Could you check a few things on this model? Use its own coordinates, in mm. Face numbers are marked on the shaded views. A direction names the side the tool comes from. Give positions to 0.01 mm unless a question says otherwise; leave off trailing zeros. Write each loop counter-clockwise with the first axis right and the second up, starting at its lowest first coordinate (ties: lowest second). Pieces come first, ordered by that corner, then holes. Notation, with made-up numbers: M -0.75,10.5 L 12.25,10.5 A11 ccw 12.25,14.5 Z; hole C -32.5,71.25 d8. An arc over 180 degrees is marked long. One line per item, written item: value.
```python
from build123d import *

# Parameters (mm, degrees)
BOSS_EXTRUDE2_DEPTH = 25.4
CUT_EXTRUDE7_START  = -1
SKETCH5_5_R         = 1.89865
CUT_EXTRUDE7_DEPTH  = 11.8425
SKETCH8_R           = 5.70865
SKETCH8_R_2         = 1.89865
BOSS_EXTRUDE4_DEPTH = 5.08
CUT_EXTRUDE8_START  = 5.08
SKETCH8_3_R         = 5.70865
SKETCH8_3_R_2       = 1.89865
CUT_EXTRUDE8_DEPTH  = 5.7625001
CUT_EXTRUDE3_DEPTH  = 26.4000001
FILLET3_R           = 1.905


with BuildPart() as part:
    # Sketch4 → Boss-Extrude2 (new body)
    with BuildSketch(Plane(origin=(-23.495, 41.0349954, 0), x_dir=(0, 0, 1), z_dir=(-1, 0, 0))):
        with BuildLine():
            ThreePointArc((0, 16.227532365), (9.8425, 0), (0, -16.227532365))
            Line((0, -16.227532365), (0, -10.16))
            ThreePointArc((0, -10.16), (4.7625, 0), (0, 10.16))
            Line((0, 10.16), (0, 16.227532365))
        make_face()
    extrude(amount=-BOSS_EXTRUDE2_DEPTH)

    # Sketch5_5 → Cut-Extrude7 (cut)
    with BuildSketch(Plane.XY.offset(CUT_EXTRUDE7_START)):
        with Locations((-10.795, 55.2907454)):
            Circle(SKETCH5_5_R)
    cut_extrude7 = extrude(amount=CUT_EXTRUDE7_DEPTH, mode=Mode.SUBTRACT)

    # Sketch8 → Boss-Extrude4 (add)
    with BuildSketch(Plane.XY):
        with Locations((-10.795, 55.2907454)):
            Circle(SKETCH8_R)
        with Locations((-10.795, 55.2907454)):
            Circle(SKETCH8_R_2, mode=Mode.SUBTRACT)
    boss_extrude4 = extrude(amount=BOSS_EXTRUDE4_DEPTH)

    # Sketch8_3 → Cut-Extrude8 (cut, through all)
    with BuildSketch(Plane.XY.offset(CUT_EXTRUDE8_START)):
        with Locations((-10.795, 55.2907454)):
            Circle(SKETCH8_3_R)
        with Locations((-10.795, 55.2907454)):
            Circle(SKETCH8_3_R_2, mode=Mode.SUBTRACT)
    cut_extrude8 = extrude(amount=CUT_EXTRUDE8_DEPTH, mode=Mode.SUBTRACT)

    # Mirror1: Cut-Extrude7, Boss-Extrude4, Cut-Extrude8 across plane
    add(cut_extrude7.mirror(Plane.ZX.offset(41.0349954)), mode=Mode.SUBTRACT)
    add(boss_extrude4.mirror(Plane.ZX.offset(41.0349954)))
    add(cut_extrude8.mirror(Plane.ZX.offset(41.0349954)), mode=Mode.SUBTRACT)

    # Sketch4_3 → Cut-Extrude3 (cut, through all)
    with BuildSketch(Plane(origin=(-23.495, 41.0349954, 0), x_dir=(0, 0, 1), z_dir=(-1, 0, 0))):
        with BuildLine():
            ThreePointArc((0, 10.16), (4.7625, 0), (0, -10.16))
            Line((0, -10.16), (0, 10.16))
        make_face()
    extrude(amount=-CUT_EXTRUDE3_DEPTH, mode=Mode.SUBTRACT)

    # Fillet3
    fillet3_edges = [part.edges().sort_by_distance(p)[0] for p in [
        (1.905, 41.0349954, 9.8425),
        (-23.495, 41.0349954, 9.8425),
    ]]
    fillet(fillet3_edges, radius=FILLET3_R)


solid = part.part
```
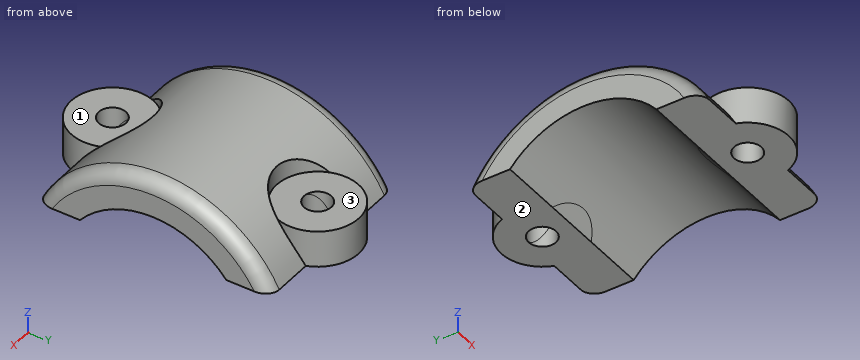
1) Please list where these lines run through material, in increasing order: L1, parallel to Z at x = -12.25, y = 29.5; L2, parallel to Y at x = -7.5, z = 3.5; L3, parallel to Y at x = 0.25, z = 1. Write a range as from..to.
Outcome:
L1: z = 0..5.08
L2: y = 22.12..35.4, 46.67..59.95
L3: y = 25.39..31.8, 50.27..56.68
2) I'm going to push flat-ended pins straight in: pin 1 (5.5 mm diameter, centred on x = -9, y = 28.5, fed in from +Z); pin 2 (2.5 mm diameter, centred on x = -10.8, y = 55.29, fed in from +Z); pin 3 (1.5 mm diameter, centred on x = -2.5, z = 1.5, fed in from +Y); pin 4 (4 mm diameter, centred on x = -15, z = 8.5, fed in from +Y). Where does each tip first touch, or does it pass through?
Outcome:
pin 1: stops at z = 5.08
pin 2: passes through
pin 3: stops at y = 56.85
pin 4: stops at y = 51.57
3) If we section it at A-A, the plane z = 3.5: Give the number of separate pieces and of enclosed holes in the cut face, then the cut area to 3 significant figures.
Outcome:
separate pieces: 2
enclosed holes: 2
area: 502 mm^2
4) If we section it at D-D, the plane x = -13.75: Write out the boundary of the cut face in (y, z) (3 decimals).
Outcome:
outline: M 21.895,0 L 30.875,0 A13.219 cw 51.195,0 L 60.175,0 L 60.175,5.08 L 50.406,5.08 L 50.406,7.261 A18.299 ccw 31.664,7.261 L 31.664,5.08 L 21.895,5.08 Z
5) On a 3-axis mill with a long thin cutter (end or side, diameter ignored), from which of +Z, -Z, +X, -X, +Y, -Y can I reach the whole of each face in a straight line? I mean the marked faces 1, 2 and 3. Say none if no direction works.
Outcome:
face 1: +Z, -Y
face 2: -Z, +X, -X, +Y, -Y
face 3: +Z, +Y
6) If we section it at B-B, the plane x = -8.5: Write out the boundary of the cut face in (y, z) (3 decimals), then the cut area to 3 significant figures.
Outcome:
outline: M 21.552,0 L 30.875,0 A13.219 cw 51.195,0 L 60.518,0 L 60.518,5.08 L 50.064,5.08 L 50.064,7.46 A18.299 ccw 32.006,7.46 L 32.006,5.08 L 21.552,5.08 Z
area: 203 mm^2
7) If we section it at C-C, the plane x = -20.5: Write out the boundary of the cut face in (y, z) (3 decimals).
Outcome:
outline: M 24.807,0 L 30.875,0 A13.219 cw 51.195,0 L 57.263,0 A18.299 ccw Z
